Geometry: final body of the model. Coordinates: model frame, mm. A direction names the side the tool comes from. Coordinates: 2 decimals unless noted, no trailing zeros. Loops run counter-clockwise (first coordinate to the right, second up) from the corner with the lowest first, then second, coordinate; pieces in that order, holes last. Notation, with made-up numbers: (-26, 45) - (-18, 45) arc R8 ccw to (-18, 54) - close; hole circle Ø5 at (22, 39.25). An arc over 180 degrees is marked (long way). Return JSON: item names as keys, results as strings.
from build123d import *

# Parameters (mm, degrees)
F1_DEPTH  = 25.4
F1_FACE_W = 12.7
F1_FACE_H = 25.4


with BuildPart() as f1:
    # F0 (on Front) → F1 (new body)
    with BuildSketch(Plane.XZ):
        with BuildLine():
            Line((-24.13, 0), (-25.4, 0))
            ThreePointArc((-25.4, 0), (-25.3920562907, -0.6351986549), (-25.3682301314, -1.27))
            Line((-25.3682301314, -1.27), (-24.0965557705, -1.27))
            ThreePointArc((-24.0965557705, -1.27), (-24.1216374936, -0.6352201423), (-24.13, 0))
        make_face()
        with BuildLine():
            ThreePointArc((-25.3682301314, -1.27), (-25.3920562907, -0.6351986549), (-25.4, 0))
            Line((-25.4, 0), (-36.83, 0))
            Line((-36.83, 0), (-36.83, -1.27))
            Line((-36.83, -1.27), (-25.3682301314, -1.27))
        make_face()
        with BuildLine():
            Line((-24.0965557705, -1.27), (-25.3682301314, -1.27))
            ThreePointArc((-25.3682301314, -1.27), (0, -25.4), (25.3682301314, -1.27))
            Line((25.3682301314, -1.27), (24.0965557705, -1.27))
            ThreePointArc((24.0965557705, -1.27), (0, -24.13), (-24.0965557705, -1.27))
        make_face()
        with BuildLine():
            Line((24.0965557705, -1.27), (25.3682301314, -1.27))
            ThreePointArc((25.3682301314, -1.27), (25.3920562907, -0.6351986549), (25.4, 0))
            Line((25.4, 0), (24.13, 0))
            ThreePointArc((24.13, 0), (24.1216374936, -0.6352201423), (24.0965557705, -1.27))
        make_face()
        with BuildLine():
            ThreePointArc((25.4, 0), (25.3920562907, -0.6351986549), (25.3682301314, -1.27))
            Line((25.3682301314, -1.27), (36.83, -1.27))
            Line((36.83, -1.27), (36.83, 0))
            Line((36.83, 0), (25.4, 0))
        make_face()
    extrude(amount=F1_DEPTH)

    # F3: sweep along a path in F2
    with BuildLine(Plane.YZ) as f3_path:
        Line((0, 0), (-47.6711578667, -33.3962440491))
    # F1_face (on face) + F1_face1 (on face) + F0 (on Front) → F3 (sweep)
    with BuildSketch(Plane(origin=(-30.48, -12.7, 0), x_dir=(1, 0, 0), z_dir=(0, 0, 1))):
        Rectangle(F1_FACE_W, F1_FACE_H)
        with Locations((60.96, 0)):
            Rectangle(F1_FACE_W, F1_FACE_H)
    with BuildSketch(Plane(origin=(1e-10, -25.4, -12.329976557), x_dir=(1, 0, 0), z_dir=(0, -1, 0))):
        with BuildLine():
            Line((-24.1300000001, 12.329976557), (-36.8300000001, 12.329976557))
            Line((-36.8300000001, 12.329976557), (-36.8300000001, 11.059976557))
            Line((-36.8300000001, 11.059976557), (-25.3682301315, 11.059976557))
            ThreePointArc((-25.3682301315, 11.059976557), (-1e-10, -13.070023443), (25.3682301313, 11.059976557))
            Line((25.3682301313, 11.059976557), (36.8299999999, 11.059976557))
            Line((36.8299999999, 11.059976557), (36.8299999999, 12.329976557))
            Line((36.8299999999, 12.329976557), (24.1299999999, 12.329976557))
            ThreePointArc((24.1299999999, 12.329976557), (-1e-10, -11.8000234431), (-24.1300000001, 12.329976557))
        make_face()
    with BuildSketch(Plane.XZ):
        with BuildLine():
            Line((-24.0965557705, -1.27), (-25.3682301314, -1.27))
            ThreePointArc((-25.3682301314, -1.27), (0, -25.4), (25.3682301314, -1.27))
            Line((25.3682301314, -1.27), (24.0965557705, -1.27))
            ThreePointArc((24.0965557705, -1.27), (0, -24.13), (-24.0965557705, -1.27))
        make_face()
    sweep(path=f3_path.line)


solid = f1.part
Item 1: Reachability of faces 1 (the face through (-24.723, -29.466, -21.913)), 2 (the face through (3.9, -47.671, -57.4)), 3 (the face through (-31.179, -11.959, 8.146)), 4 (the face through (-0.541, -12.522, -25.394)) from +Z, -Z, +X, -X, +Y, -Y: full face, straight path, thin tool, end or side. Return the list, or none.
Worked out:
{"face 1": "-X", "face 2": "-Z, +X, -X, -Y", "face 3": "-X, +Y", "face 4": "none"}
Item 2: First-contact query: pin 1 Ø1.5 at (x, y) = (32, -1) entering from -Z; pin 2 Ø20.5 at (x, z) = (0, -30) entering from -Y; pin 3 Ø14 at (x, y) = (-31, -65.5) entering from -Z. Flat tips, straight axial feed; report the tip coordinate or a pass-through.
Worked out:
{"pin 1": "z = -1.27", "pin 2": "y = -47.67", "pin 3": "z = -33.4"}
Item 3: Mould query, pull axis Z, two halves, no side actions, for faces 5 (the face through (31, -12, 0)), 6 (the face through (-3, -47.671, -40)), 7 (the face through (30.57, -37.05, -8.16)). Classes: +Z half, -Z half, draft (parallel to the pull), parting line (faces both ways), or undercut.
Worked out:
{"face 5": "undercut", "face 6": "draft", "face 7": "+Z half"}
Item 4: Section query B-B, the plane x = -26.5. Return loops of the section in (y, z).
Worked out:
{"outline": "(-73.07, -33.4) - (-47.67, -33.4) - (-1.81, -1.27) - (0, -1.27) - (0, 0) - (-23.59, 0) - (0, 16.52) - (0, 17.79) - close"}
Item 5: Section query A-A, the plane y = -57. Return loops of the section in (x, z), and give its area (3 significant figures).
Worked out:
{"outline": "(-36.83, -33.4) - (-24.13, -33.4) - (-24.13, -22.14) - (-36.83, -22.14) - close; (24.13, -33.4) - (36.83, -33.4) - (36.83, -22.14) - (24.13, -22.14) - close", "area": "286 mm^2"}
Item 6: Ray query, probe 1 along X at (y, z) = (-21.5, -4); probe 2 along Z at (x, y) = (30.5, -15); probe 3 along Z at (x, y) = (14.5, -11.5). Return the intervals inside material, ascending. Write a range as from..to.
Worked out:
{"probe 1": "-36.83..-23.17, 23.17..36.83", "probe 2": "-10.51..0, 6.02..7.29", "probe 3": "-28.91..-27.34, -20.85..-19.29, -11.12..-9.55"}
